```python
from build123d import *


with BuildPart() as part:
    # Sketch → Revolution (revolve)
    with BuildSketch(Plane.XZ):
        with BuildLine():
            Line((-50, 34.7391), (-32, -30))
            Line((-32, -30), (-30, -30))
            ThreePointArc((-6.05, -10), (-22.702813, -14.398319), (-30, -30))
            Line((-6.05, 10), (-6.05, -10))
            Line((-6.05, 10), (-11.265964, -7.547867))
            ThreePointArc((-11.265964, -7.547867), (-24.914311, -13.814151), (-31, -27.543976))
            Line((-49, 37.195124), (-31, -27.543976))
            Line((-50, 34.7391), (-49, 37.195124))
        make_face()
    revolve(axis=Axis((0, 0, 0), (0, 0, 1)))


solid = part.part
```
Geometry check sheet. Reference: the model listing, model coordinates, mm. Round coordinates to 2 decimals unless told otherwise and drop trailing zeros. Loops run counter-clockwise (first coordinate to the right, second up) from the corner with the lowest first, then second, coordinate; pieces in that order, holes last. Notation, with made-up numbers: M -6,1.5 L 14,1.5 A20 cw 14,36.5 Z; hole C -5,60.5 d9. An arc over 180 degrees is marked long. Return JSON: item names as keys, results as strings. Group by question number.
(1) Section check A-A, the plane z = 6. Enter the section's corners in (x, y).
(2) Scan lines: line 1 along Y through (x, z) = (6, -23.5); line 2 along Y through (x, z) = (0, 5.25); line 3 along X through (y, z) = (0, -3). Record each from-to range of solid material in increasing order. Write a range as [from, to].
(3) Mould release check, pull along X, two halves, no side actions. Record for faces 1 (the face through (-37.079, -11.677, -5.277)), 2 (the face through (8.21, 36.973, -2.821)), 3 (the face through (-9, -29, -30)): pulls with the +X half, pulls with the -X half, needs draft (parallel to the pull), parting line crosses it, or undercut.
(4) Section check B-B, the plane z = -1.5. Enter the section's corners in (x, y), and give its area (3 significant figures).
(5) Go/stop test with flat-tipped pins: pin 1 (10 mm diameter, centred on x = -4, z = 24, fed in from +Y); pin 2 (10 mm diameter, centred on y = -14.5, z = -14.5, fed in from -X); pin 3 (1 mm diameter, centred on x = 5.5, z = -17.5, fed in from -Y). Record where each tip stops, or that it passes through.
Data:
{
 "1": {"outline": "C 0,0 d84.02; C 0,0 d14.48; hole C 0,0 d80.65; hole C 0,0 d12.1"},
 "2": {"line 1": "[-33.27, -31.56], [-29.78, -28.3], [28.3, 29.78], [31.56, 33.27]", "line 2": "[-41.8, -40.12], [-7.46, -6.05], [6.05, 7.46], [40.12, 41.8]", "line 3": "[-39.51, -37.82], [-9.91, -6.05], [6.05, 9.91], [37.82, 39.51]"},
 "3": {"face 1": "parting line crosses it", "face 2": "undercut", "face 3": "needs draft"},
 "4": {"outline": "C 0,0 d79.85; C 0,0 d18.94; hole C 0,0 d76.48; hole C 0,0 d12.1", "area": "580 mm²"},
 "5": {"pin 1": "y = 48.28", "pin 2": "x = -35.65", "pin 3": "y = -35.21"}
}
